Verification items for the finished model (mm, model axes). A direction names the side the tool comes from. Round coordinates to 2 decimals unless told otherwise and drop trailing zeros. Write each loop counter-clockwise with the first axis right and the second up, starting at its lowest first coordinate (ties: lowest second). Pieces come first, ordered by that corner, then holes. Notation, with made-up numbers: (87.5, 54.25) -> (105.5, 54.25) arc R28 cw to (105.5, 86.25) -> close; hole circle Ø10 at (50, 44). An arc over 180 degrees is marked (long way). Use CSV: the item, a comma, the result in double quotes.
```python
from build123d import *

# Parameters (mm, degrees)
F1_DEPTH = 88.9
F3_D     = 6.35
F4_SIZE  = 5.08
F6_D     = 6.35


with BuildPart() as f1:
    # F0 (on Front) → F1 (new body)
    with BuildSketch(Plane.XZ):
        Polygon((0, 38.6051108942), (0, 0), (6.35, 0), (6.35, 32.2551108942), (63.5, 32.2551108942), (63.5, 38.6051108942), align=None)
    extrude(amount=F1_DEPTH)

    # F3 (through all)
    with Locations(Plane(origin=(0, 0, 0), x_dir=(0, 1, 0), z_dir=(-1, 0, 0))):
        with Locations((-76.2, -12.7), (-12.7, -12.7)):
            Hole(F3_D / 2)

    # F4
    f4_edges = [f1.edges().sort_by_distance(p)[0] for p in [
        (63.5, 0, 35.430111),
        (63.5, -88.9, 35.430111),
        (3.175, -88.9, 0),
        (3.175, 0, 0),
    ]]
    chamfer(f4_edges, length=F4_SIZE)

    # F6 (through all)
    with Locations(Plane.XY.offset(38.6051108942)):
        with Locations((25.4, -11.1252), (11.1252, -11.1252), (11.1252, -77.8002), (25.4, -77.8002)):
            Hole(F6_D / 2)


solid = f1.part
```
Q1. Go/stop test with flat-tipped pins: P1, Ø10, axis at x = 46, y = -65, coming from the -Z side; P2, Ø8.5, axis at y = -12.7, z = 12.7, coming from the -X side; P3, Ø8, axis at y = -28.5, z = 4, coming from the +X side. Record where each tip stops, or that it passes through.
Filled in:
P1,"z = 32.26"
P2,"x = 0"
P3,"x = 6.35"
Q2. Material ranges on L1, parallel to Y at x = 25.4, z = 34.5; L2, parallel to Y at x = 25, z = 35; L3, parallel to Z at x = 31, y = -15.5, recorded low to high.
Filled in:
L1,"-88.9 to -80.98, -74.63 to -14.3, -7.95 to 0"
L2,"-88.9 to -80.95, -74.65 to -14.27, -7.98 to 0"
L3,"32.26 to 38.61"
Q3. Section check D-D (y = -21). Record the cut outline in (x, z).
Filled in:
outline,"(0, 0) -> (6.35, 0) -> (6.35, 32.26) -> (63.5, 32.26) -> (63.5, 38.61) -> (0, 38.61) -> close"
Q4. Section check B-B (z = 12.7). Record the cut outline in (x, y) (3 decimals).
Filled in:
outline,"(0, -88.9) -> (6.35, -88.9) -> (6.35, -79.375) -> (0, -79.375) -> close; (0, -73.025) -> (6.35, -73.025) -> (6.35, -15.875) -> (0, -15.875) -> close; (0, -9.525) -> (6.35, -9.525) -> (6.35, 0) -> (0, 0) -> close"
Q5. Access from +Z, -Z, +X, -X, +Y, -Y to the whole of each face (thin tool, end or side, straight path). Record for faces 5 (the flat face through (32, -44, 38.605)), 6 (the flat face through (35, -44, 32.255)).
Filled in:
face 5,"+Z, +X, -X, +Y, -Y"
face 6,"-Z, +X, +Y, -Y"
Q6. Mould release check, pull along X, two halves, no side actions. Record for faces 1 (the cylindrical face through (23.9, -80.6, 35.4)), 2 (the flat face through (61, -86.32, 35.39)), 3 (the cylindrical face through (11.81, -80.9, 35.39)), 4 (the flat face through (23, 0, 33)): released by +X, released by -X, zero draft, split by the parting line, or undercut.
Filled in:
face 1,"undercut"
face 2,"released by +X"
face 3,"undercut"
face 4,"zero draft"
Q7. Section check C-C (y = -76.2). Record the cut outline in (x, z) (3 decimals), plus the area to 3 significant figures.
Filled in:
outline,"(0, 0) -> (6.35, 0) -> (6.35, 9.525) -> (0, 9.525) -> close; (0, 15.875) -> (6.35, 15.875) -> (6.35, 32.255) -> (8.383, 32.255) -> (8.383, 38.605) -> (0, 38.605) -> close; (13.867, 32.255) -> (22.658, 32.255) -> (22.658, 38.605) -> (13.867, 38.605) -> close; (28.142, 32.255) -> (63.5, 32.255) -> (63.5, 38.605) -> (28.142, 38.605) -> close"
area,"498 mm²"
Q8. Section check A-A (x = 25.4). Record the cut outline in (y, z).
Filled in:
outline,"(-88.9, 32.26) -> (-80.98, 32.26) -> (-80.98, 38.61) -> (-88.9, 38.61) -> close; (-74.63, 32.26) -> (-14.3, 32.26) -> (-14.3, 38.61) -> (-74.63, 38.61) -> close; (-7.95, 32.26) -> (0, 32.26) -> (0, 38.61) -> (-7.95, 38.61) -> close"
